Job drawing, mm, ordinate dimensions from the low corner. One solid piece. Give positions to 0.01 mm unless a question says otherwise; leave off trailing zeros. Loops run counter-clockwise (first coordinate to the right, second up) from the corner with the lowest first, then second, coordinate; pieces in that order, holes last.
Item 1: Saw through at C-C on y = 4. Give the cut face in (x, z).
Item 2: Probe probe 1 along Y at (x, z) = (1.85, 39.5); probe 2 along X at (y, z) = (8.5, 6.5). List the from-to ranges inside material, lowest first.
Item 3: Drop flat-ended pins along their axis: P1, Ø3, axis at x = 26.5, z = 16.5, coming from the +Y side; P2, Ø23, axis at y = 28, z = 25, coming from the +X side. Give the stop position or say it passes through.
Item 4: Saw through at B-B on y = 28. Give the cut face in (x, z).
Item 5: Mould opens along X. For the marked faces 1, 2 and 3 say: released by +X, released by -X, zero draft, split by the parting line, or undercut.
Item 6: Saw through at A-A on z = 25. Give the cut face in (x, y), plus the area to 3 significant figures.
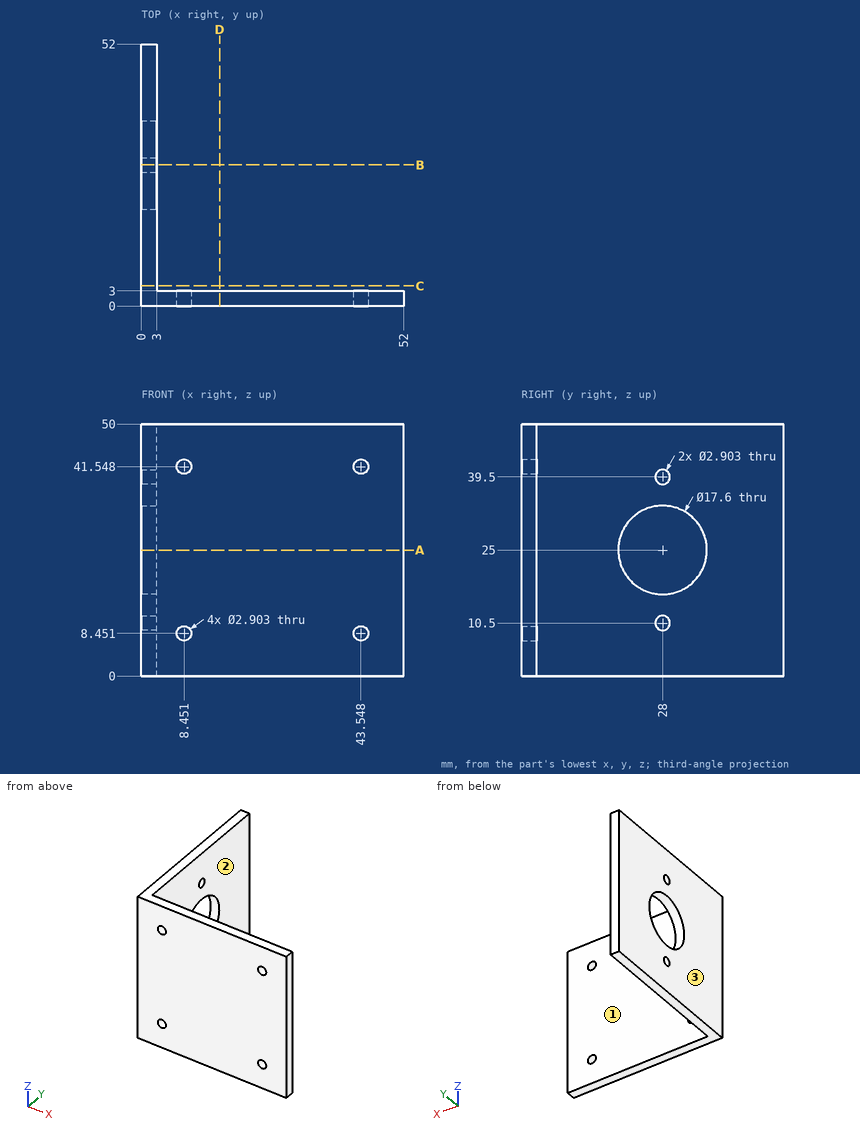
Results below:
1. outline: (0, 0) - (3, 0) - (3, 50) - (0, 50) - close
2. probe 1: y = 0 to 26.55, 29.45 to 52
2. probe 2: x = 0 to 3
3. P1: stops at y = 3
3. P2: stops at x = 3
4. outline: (0, 0) - (3, 0) - (3, 9.05) - (0, 9.05) - close; (0, 11.95) - (3, 11.95) - (3, 16.2) - (0, 16.2) - close; (0, 33.8) - (3, 33.8) - (3, 38.05) - (0, 38.05) - close; (0, 40.95) - (3, 40.95) - (3, 50) - (0, 50) - close
5. face 1: zero draft
5. face 2: released by +X
5. face 3: released by -X
6. outline: (0, 0) - (52, 0) - (52, 3) - (3, 3) - (3, 19.2) - (0, 19.2) - close; (0, 36.8) - (3, 36.8) - (3, 52) - (0, 52) - close
6. area: 250 mm2
